Read the model definition and answer for the solid it produces. Units are mm, in the model's axes. A direction names the side the tool comes from. Give positions to 0.01 mm unless a question says otherwise; leave off trailing zeros. Loops run counter-clockwise (first coordinate to the right, second up) from the corner with the lowest first, then second, coordinate; pieces in that order, holes last. Notation, with made-up numbers: (49.5, 4) - (83.5, 4) arc R21 ccw to (83.5, 39) - close; hole circle Ø11 at (-30.5, -4). An arc over 180 degrees is marked (long way). Use a Markdown table: item, result. Add a question column.
Item 1: A cutting plane is placed at A-A (x = 41.91). Determine the outline of the cut face in (y, z) (3 decimals), plus the area to 3 significant figures.
Item 2: Each of these flat-tipped pins is pushed along its axis until it touches: P1, Ø3.5, axis at x = 10.16, z = -16.891, coming from the +Y side; P2, Ø1, axis at x = 33, z = -18.5, coming from the +Y side; P3, Ø1.5, axis at x = 39.5, z = -17, coming from the +Y side (3 decimals); P4, Ø2.5, axis at x = 27, z = -15, coming from the -Y side (3 decimals). Where does it stop, or does it pass through?
Item 3: For a pull along X with two mould halves and no side action, classify faces 4 (the face through (7, 0, -17)), 5 (the face through (54.61, 5, -17)), 6 (the face through (52.07, 8, -17)), 7 (the face through (45.944, 3.47, -18.161)) as +X half, -X half, draft (parallel to the pull), parting line (faces both ways), or undercut.
Item 4: A cutting plane is placed at B-B (y = 7.75). Determine the outline of the cut face in (x, z) (3 decimals), plus the area to 3 significant figures.
Item 5: A cutting plane is placed at D-D (x = 31.5). Determine the outline of the cut face in (y, z), plus the area to 3 significant figures.
Item 6: Which of the six approach directions +Z, -Z, +X, -X, +Y, -Y give full straight-line access (tool end or side, diameter ignored) to faces 1 (the face through (0.724, 7.656, -0.764)), 2 (the face through (39, 0, -17)), 3 (the face through (26, 1.905, -17))?
Item 7: A cutting plane is placed at C-C (z = -11). Determine the outline of the cut face in (x, y) (3 decimals), plus the area to 3 significant figures.
Item 8: Consider probe 1 along X at (y, z) = (8.5, -7); probe 2 along Z at (x, y) = (41.91, 3.15); probe 3 along Z at (x, y) = (10.16, 0.6) (3 decimals). Determine where each line is inside the solid, lowest interval first. Write a range as [from, to].
from build123d import *

# Parameters (mm, degrees)
SKETCH1_W           = 22.225
SKETCH1_H           = 33.782
SKETCH1_R           = 4.2291
SKETCH1_R_2         = 2.286
BOSS_EXTRUDE1_DEPTH = 1.905
BOSS_EXTRUDE2_START = 1.905
SKETCH1_3_W         = 22.225
SKETCH1_3_H         = 33.782
SKETCH1_3_R         = 4.2291
SKETCH1_3_W_2       = 7.62
BOSS_EXTRUDE2_DEPTH = 3.175
BOSS_EXTRUDE3_START = 5.08
BOSS_EXTRUDE3_DEPTH = 5.08
FILLET1_R           = 2.54
FILLET2_R           = 2.54


with BuildPart() as part:
    # Sketch1 → Boss-Extrude1 (new body)
    with BuildSketch(Plane(origin=(0, 0, 0), x_dir=(1, 0, 0), z_dir=(0, 1, 0))):
        Polygon((22.225, 36.322), (-2.54, 36.322), (-2.54, -2.54), (22.225, -2.54), (22.225, 0), (0, 0), (0, 33.782), (22.225, 33.782), align=None)
        with Locations((11.1125, 16.891)):
            Rectangle(SKETCH1_W, SKETCH1_H)
        with Locations((10.16, 16.891)):
            Circle(SKETCH1_R, mode=Mode.SUBTRACT)
        with Locations((10.16, 16.891)):
            Circle(SKETCH1_R)
        with Locations((10.16, 16.891)):
            Circle(SKETCH1_R_2, mode=Mode.SUBTRACT)
        with Locations((40.9575, 16.891)):
            Rectangle(SKETCH1_W, SKETCH1_H)
        with Locations((41.91, 16.891)):
            Circle(SKETCH1_R, mode=Mode.SUBTRACT)
        with Locations((41.91, 16.891)):
            Circle(SKETCH1_R)
        with Locations((41.91, 16.891)):
            Circle(SKETCH1_R_2, mode=Mode.SUBTRACT)
        Polygon((54.61, 36.322), (29.845, 36.322), (29.845, 33.782), (52.07, 33.782), (52.07, 0), (29.845, 0), (29.845, -2.54), (54.61, -2.54), align=None)
    extrude(amount=BOSS_EXTRUDE1_DEPTH)

    # Sketch1_3 → Boss-Extrude2 (add)
    with BuildSketch(Plane(origin=(0, 0, 0), x_dir=(1, 0, 0), z_dir=(0, 1, 0)).offset(BOSS_EXTRUDE2_START)):
        with Locations((11.1125, 16.891)):
            Rectangle(SKETCH1_3_W, SKETCH1_3_H)
        with Locations((10.16, 16.891)):
            Circle(SKETCH1_3_R, mode=Mode.SUBTRACT)
        with Locations((40.9575, 16.891)):
            Rectangle(SKETCH1_3_W, SKETCH1_3_H)
        with Locations((41.91, 16.891)):
            Circle(SKETCH1_3_R, mode=Mode.SUBTRACT)
        with Locations((26.035, 16.891)):
            Rectangle(SKETCH1_3_W_2, SKETCH1_3_H)
        Polygon((22.225, 36.322), (-2.54, 36.322), (-2.54, -2.54), (22.225, -2.54), (22.225, 0), (0, 0), (0, 33.782), (22.225, 33.782), align=None)
        Polygon((54.61, 36.322), (29.845, 36.322), (29.845, 33.782), (52.07, 33.782), (52.07, 0), (29.845, 0), (29.845, -2.54), (54.61, -2.54), align=None)
    extrude(amount=BOSS_EXTRUDE2_DEPTH)

    # Sketch1_4 → Boss-Extrude3 (add)
    with BuildSketch(Plane(origin=(0, 0, 0), x_dir=(1, 0, 0), z_dir=(0, 1, 0)).offset(BOSS_EXTRUDE3_START)):
        Polygon((22.225, 36.322), (-2.54, 36.322), (-2.54, -2.54), (22.225, -2.54), (22.225, 0), (0, 0), (0, 33.782), (22.225, 33.782), align=None)
        Polygon((54.61, 36.322), (29.845, 36.322), (29.845, 33.782), (52.07, 33.782), (52.07, 0), (29.845, 0), (29.845, -2.54), (54.61, -2.54), align=None)
    extrude(amount=BOSS_EXTRUDE3_DEPTH)

    # Fillet1
    fillet1_edges = [part.edges().sort_by_distance(p)[0] for p in [
        (-2.54, 5.08, 2.54),
        (-2.54, 5.08, -36.322),
        (54.61, 5.08, 2.54),
        (54.61, 5.08, -36.322),
        (0, 7.62, 0),
        (0, 7.62, -33.782),
        (52.07, 7.62, -33.782),
        (52.07, 7.62, 0),
    ]]
    fillet(fillet1_edges, radius=FILLET1_R)

    # Fillet2
    fillet2_edges = [part.edges().sort_by_distance(p)[0] for p in [
        (26.035, 1.905, -33.782),
        (26.035, 1.905, 0),
    ]]
    fillet(fillet2_edges, radius=FILLET2_R)


solid = part.part
Geometry says:
| question | item | result |
|---|---|---|
| 1 | outline | (0, -36.322) - (10.16, -36.322) - (10.16, -33.782) - (5.08, -33.782) - (5.08, -21.12) - (1.905, -21.12) - (1.905, -19.177) - (0, -19.177) - close; (0, -14.605) - (1.905, -14.605) - (1.905, -12.662) - (5.08, -12.662) - (5.08, 0) - (10.16, 0) - (10.16, 2.54) - (0, 2.54) - close |
| 1 | area | 188 mm² |
| 2 | P1 | through |
| 2 | P2 | y = 5.08 |
| 2 | P3 | y = 1.905 |
| 2 | P4 | y = 1.905 |
| 3 | face 4 | draft |
| 3 | face 5 | +X half |
| 3 | face 6 | undercut |
| 3 | face 7 | undercut |
| 4 | outline | (-2.54, -33.782) arc R2.54 ccw to (0, -36.322) - (22.225, -36.322) - (22.225, -33.782) - (2.54, -33.782) arc R2.54 cw to (0, -31.242) - (0, -2.54) arc R2.54 cw to (2.54, 0) - (22.225, 0) - (22.225, 2.54) - (0, 2.54) arc R2.54 ccw to (-2.54, 0) - close; (29.845, -36.322) - (52.07, -36.322) arc R2.54 ccw to (54.61, -33.782) - (54.61, 0) arc R2.54 ccw to (52.07, 2.54) - (29.845, 2.54) - (29.845, 0) - (49.53, 0) arc R2.54 cw to (52.07, -2.54) - (52.07, -31.242) arc R2.54 cw to (49.53, -33.782) - (29.845, -33.782) - close |
| 4 | area | 423 mm² |
| 5 | outline | (0, -36.32) - (10.16, -36.32) - (10.16, -33.78) - (5.08, -33.78) - (5.08, 0) - (10.16, 0) - (10.16, 2.54) - (0, 2.54) - close |
| 5 | area | 223 mm² |
| 6 | face 1 | +Y |
| 6 | face 2 | +Z, -Z, +X, -X, -Y |
| 6 | face 3 | +Z, -Z, -Y |
| 7 | outline | (-2.54, 0) - (22.225, 0) - (22.225, 1.905) - (29.845, 1.905) - (29.845, 0) - (54.61, 0) - (54.61, 10.16) - (52.07, 10.16) - (52.07, 5.08) - (0, 5.08) - (0, 10.16) - (-2.54, 10.16) - close |
| 7 | area | 302 mm² |
| 8 | probe 1 | [-2.54, 0], [52.07, 54.61] |
| 8 | probe 2 | [-36.32, -21.12], [-12.66, 2.54] |
| 8 | probe 3 | [-36.322, -19.177], [-14.605, 2.54] |
